from build123d import *
from build123d.topology import SkipClean

# Parameters (mm, degrees)
SKETCH2_R           = 5.1000000000000005
BOSS_EXTRUDE1_DEPTH = 1
SKETCH3_R           = 5.1000000000000005
SKETCH3_R_2         = 4.3
BOSS_EXTRUDE2_DEPTH = 12
CUT_EXTRUDE2_DEPTH  = 1
SKETCH7_R           = 7.5
SKETCH7_R_2         = 5.1000000000000005
BOSS_EXTRUDE4_DEPTH = 2


with BuildPart() as part:
    # Sketch2 → Boss-Extrude1 (new body)
    with BuildSketch(Plane(origin=(0, 0, 0), x_dir=(1, 0, 0), z_dir=(0, 1, 0))):
        with Locations(Location((0, 0, 0), (0, 0, 270))):
            Circle(SKETCH2_R)
    extrude(amount=BOSS_EXTRUDE1_DEPTH)

    # Sketch3 → Boss-Extrude2 (add)
    with BuildSketch(Plane(origin=(0, 1, 0), x_dir=(1, 0, 0), z_dir=(0, 1, 0))):
        with Locations(Location((0, 0, 0), (0, 0, 270))):
            Circle(SKETCH3_R)
        with Locations(Location((0, 0, 0), (0, 0, 270))):
            Circle(SKETCH3_R_2, mode=Mode.SUBTRACT)
    extrude(amount=BOSS_EXTRUDE2_DEPTH)

    # Sketch6 → Cut-Extrude2 (cut)
    with BuildSketch(Plane(origin=(0, 1, 0), x_dir=(1, 0, 0), z_dir=(0, 1, 0))):
        with BuildLine():
            ThreePointArc((-1.767766952966369, 1.7677669529663689), (-2.1650635094610977, 1.2499999999999991), (-2.4148145657226716, 0.6470476127562977))
            Line((-2.4148145657226716, 0.6470476127562977), (-3.1875552267539264, 0.8541028488383131))
            ThreePointArc((-3.1875552267539264, 0.8541028488383131), (-2.857883832488649, 1.6499999999999986), (-2.333452377915607, 2.3334523779156067))
            Line((-2.333452377915607, 2.3334523779156067), (-1.767766952966369, 1.7677669529663689))
        make_face()
        with BuildLine():
            ThreePointArc((2.414814565722671, 0.6470476127563006), (2.1650635094610964, 1.2500000000000004), (1.7677669529663664, 1.7677669529663707))
            Line((1.7677669529663664, 1.7677669529663707), (2.3334523779156044, 2.3334523779156093))
            ThreePointArc((2.3334523779156044, 2.3334523779156093), (2.8578838324886475, 1.650000000000001), (3.1875552267539264, 0.8541028488383169))
            Line((3.1875552267539264, 0.8541028488383169), (2.414814565722671, 0.6470476127563006))
        make_face()
        with BuildLine():
            ThreePointArc((1.7677669529663684, -1.76776695296637), (2.1650635094610973, -1.2499999999999993), (2.414814565722671, -0.6470476127562991))
            Line((2.414814565722671, -0.6470476127562991), (3.1875552267539264, -0.8541028488383147))
            ThreePointArc((3.1875552267539264, -0.8541028488383147), (2.857883832488649, -1.6499999999999992), (2.3334523779156067, -2.333452377915608))
            Line((2.3334523779156067, -2.333452377915608), (1.7677669529663684, -1.76776695296637))
        make_face()
        with BuildLine():
            ThreePointArc((-0.6470476127563032, -2.4148145657226703), (7.1e-16, -2.5), (0.6470476127563044, -2.41481456572267))
            Line((0.6470476127563044, -2.41481456572267), (0.8541028488383218, -3.187555226753924))
            ThreePointArc((0.8541028488383218, -3.187555226753924), (9.3e-16, -3.3000000000000003), (-0.8541028488383201, -3.187555226753925))
            Line((-0.8541028488383201, -3.187555226753925), (-0.6470476127563032, -2.4148145657226703))
        make_face()
        with BuildLine():
            ThreePointArc((-2.414814565722671, -0.6470476127563016), (-2.1650635094610964, -1.250000000000001), (-1.7677669529663664, -1.7677669529663715))
            Line((-1.7677669529663664, -1.7677669529663715), (-2.3334523779156036, -2.33345237791561))
            ThreePointArc((-2.3334523779156036, -2.33345237791561), (-2.857883832488647, -1.6500000000000012), (-3.1875552267539256, -0.8541028488383182))
            Line((-3.1875552267539256, -0.8541028488383182), (-2.414814565722671, -0.6470476127563016))
        make_face()
        with BuildLine():
            ThreePointArc((0.6470476127563035, 2.4148145657226703), (-4e-16, 2.5), (-0.6470476127563042, 2.41481456572267))
            Line((-0.6470476127563042, 2.41481456572267), (-0.8541028488383214, 3.187555226753924))
            ThreePointArc((-0.8541028488383214, 3.187555226753924), (-5.3e-16, 3.3000000000000003), (0.8541028488383205, 3.187555226753925))
            Line((0.8541028488383205, 3.187555226753925), (0.6470476127563035, 2.4148145657226703))
        make_face()
    extrude(amount=-CUT_EXTRUDE2_DEPTH, mode=Mode.SUBTRACT)

    # Sketch7 → Boss-Extrude4 (add)
    with BuildSketch(Plane(origin=(0, 6, 0), x_dir=(1, 0, 0), z_dir=(0, 1, 0))):
        with Locations(Location((0, 0, 0), (0, 0, 270))):
            Circle(SKETCH7_R)
        with Locations(Location((0, 0, 0), (0, 0, 270))):
            Circle(SKETCH7_R_2, mode=Mode.SUBTRACT)
    extrude(amount=BOSS_EXTRUDE4_DEPTH)

    # Sketch8 → Revolve1 (revolve)
    with SkipClean():  # the faces are left unmerged after this step: merging them gives an invalid solid
        with BuildSketch(Plane(origin=(0, 0, 0), x_dir=(0, 0, -1), z_dir=(1, 0, 0)), mode=Mode.PRIVATE) as revolve1_sk:
            with BuildLine():
                ThreePointArc((2.0000000000000013, -11.651866191443357), (1.0373712321606319, -11.240497250076075), (-8.376e-14, -11.099999999999998))
                Line((0, -11.099999999999998), (0, -15))
                Line((0, -15), (0, -18.9))
                ThreePointArc((-7.2e-16, -18.900000000000002), (2.7577164466275366, -17.757716446627537), (3.9000000000000026, -15.000000000000002))
                ThreePointArc((3.9000000000000026, -15), (3.391902121229328, -13.075162344507984), (2.0000000000000013, -11.651866191443357))
            make_face()
            with BuildLine():
                Line((0, -15), (0, -11.099999999999998))
                ThreePointArc((-8.376e-14, -11.099999999999998), (-1.0373712321607116, -11.240497250076096), (-2.000000000000001, -11.651866191443355))
                ThreePointArc((-2.000000000000001, -11.651866191443355), (-3.759502749923914, -16.03737123216067), (-7.2e-16, -18.900000000000002))
                Line((0, -18.9), (0, -15))
            make_face()
            with BuildLine():
                Line((0, -11.099999999999998), (0, 0))
                Line((0, 0), (-2, 0))
                Line((-2, 0), (-2, -11.651866191443357))
                ThreePointArc((-2.000000000000001, -11.651866191443355), (-1.0373712321607116, -11.240497250076096), (-8.376e-14, -11.099999999999998))
            make_face()
        revolve(revolve1_sk.sketch.rotate(Axis((0, 0, 0), (0, -1, 0)), 180), axis=Axis((0, 0, 0), (0, -1, 0)))


solid = part.part
Read the model definition and answer for the solid it produces. Units are mm, in the model's axes. A direction names the side the tool comes from. Give positions to 0.01 mm unless a question says otherwise; leave off trailing zeros. Write each loop counter-clockwise with the first axis right and the second up, starting at its lowest first coordinate (ties: lowest second). Pieces come first, ordered by that corner, then holes. Notation, with made-up numbers: (-11, -8.5) - (0, -8.5) arc R17 ccw to (0, 24.5) - close; hole circle Ø7 at (-15, -13). An arc over 180 degrees is marked (long way). Answer in a Markdown table with one row per item. Add a question column.
Item 1: Find the intervals of material crossed by L1, parallel to X at y = 10.25, z = 0; L2, parallel to Y at x = -6.5, z = 0.5; L3, parallel to X at y = 7.75, z = 0, in increasing order.
Item 2: Determine the mould class of faces 1 (the face through (-2.16, 0.51, -1.26)), 2 (the face through (-5, 8, 2)), 3 (the face through (-2, -6, 0)) for opening direction Y: pulls with the +Y half, pulls with the -Y half, needs draft (parallel to the pull), parting line crosses it, or undercut.
Item 3: Section C-C, the plane y = -9 is taken. Write down the section's boundary in (x, z), and give its area (3 significant figures).
Item 4: Section A-A, the plane z = -1.25 is taken. Write down the section's boundary in (x, y), and give its area (3 significant figures).
Item 5: Flat-ended cylindrical pins translate along their axes: P1, Ø3, axis at x = -2, z = 2, coming from the -Y side; P2, Ø1, axis at x = 5.5, z = 3.5, coming from the +Y side; P3, Ø3, axis at x = 1, y = -1, coming from the -Z side. Find the tip coordinate at first contact, or state that the pin passes through.
Item 6: A tool of negligible diameter and unlimited length cuts with its end or side. For faces 4 (the face through (-4, 13, -2)), 5 (the face through (-5, 6, 2)), 6 (the face through (0, 0.5, -2.5)), 7 (the face through (-2.2, 0, -0.1)), from which of +Z, -Z, +X, -X, +Y, -Y can it reach the whole face along a straight path? Write none if from no direction.
Item 7: Section B-B, the plane y = 3 is taken. Write down the section's boundary in (x, z), and give its area (3 significant figures).
Recorded:
| question | item | result |
|---|---|---|
| 1 | L1 | x = -5.1 to -4.3, 4.3 to 5.1 |
| 1 | L2 | y = 6 to 8 |
| 1 | L3 | x = -7.5 to -4.3, 4.3 to 7.5 |
| 2 | face 1 | needs draft |
| 2 | face 2 | pulls with the +Y half |
| 2 | face 3 | undercut |
| 3 | outline | circle Ø4 at (0, 0) |
| 3 | area | 12.6 mm2 |
| 4 | outline | (-7.4, 6) - (-4.94, 6) - (-4.94, 0) - (-3.05, 0) - (-3.05, 1) - (-4.11, 1) - (-4.11, 13) - (-4.94, 13) - (-4.94, 8) - (-7.4, 8) - close; (-2.17, 0) - (-1.56, 0) - (-1.56, -11.65) arc R3.69 ccw (long way) to (1.56, -11.65) - (1.56, 0) - (2.17, 0) - (2.17, 1) - (-2.17, 1) - close; (3.05, 0) - (4.94, 0) - (4.94, 6) - (7.4, 6) - (7.4, 8) - (4.94, 8) - (4.94, 13) - (4.11, 13) - (4.11, 1) - (3.05, 1) - close |
| 4 | area | 116 mm2 |
| 5 | P1 | stops at y = -18.67 |
| 5 | P2 | stops at y = 8 |
| 5 | P3 | stops at z = -5.1 |
| 6 | face 4 | +Z, -Z, +X, -X, +Y |
| 6 | face 5 | -Y |
| 6 | face 6 | +Y |
| 6 | face 7 | none |
| 7 | outline | circle Ø10.2 at (0, 0); hole circle Ø8.6 at (0, 0) |
| 7 | area | 23.6 mm2 |
